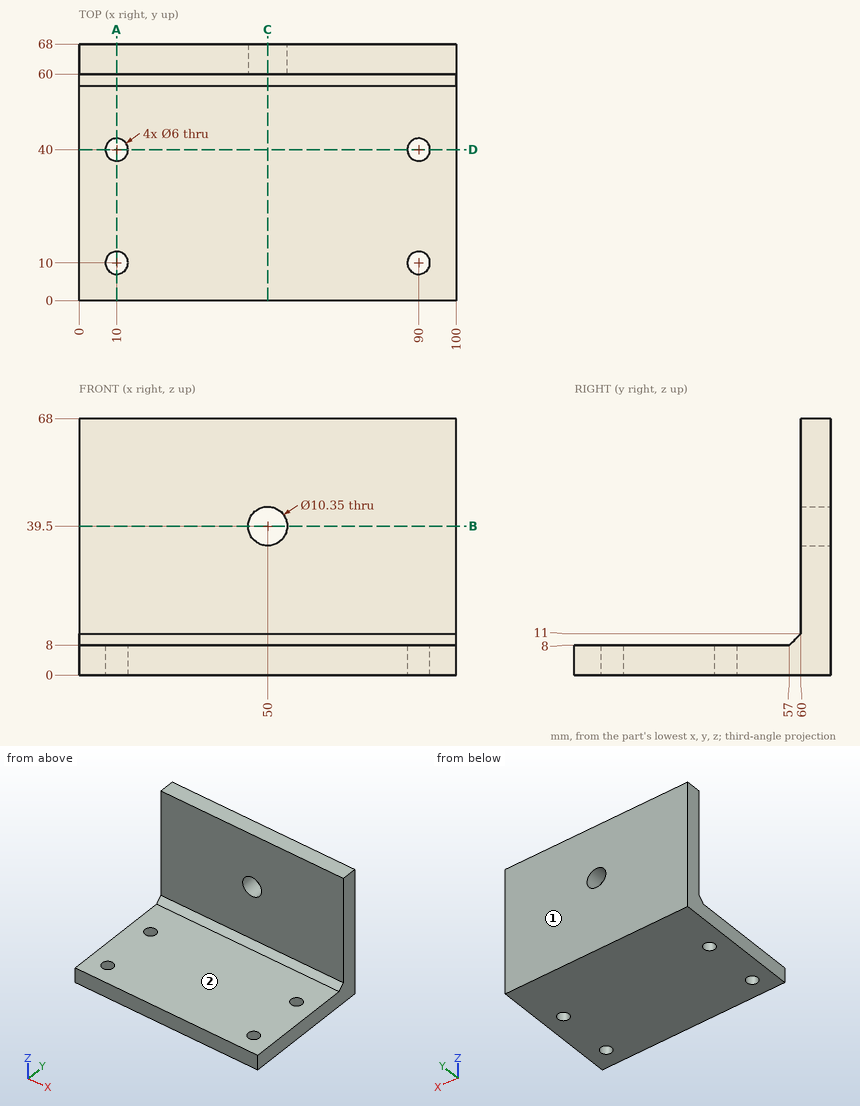
Answer from the drawing. Dimensions are ordinates in mm from the lowest x, y and z of the part. A direction names the side the tool comes from. Coordinates: 2 decimals unless noted, no trailing zeros. Write each loop counter-clockwise with the first axis right and the second up, starting at its lowest first coordinate (ties: lowest second). Pieces come first, ordered by that corner, then holes. Notation, with made-up numbers: (78.25, 62.5) - (114.25, 62.5) arc R24 cw to (114.25, 87.5) - close; hole circle Ø8 at (27, 89.25). An arc over 180 degrees is marked (long way). Return JSON: item names as keys, results as strings. Group by question number.
Q1. Find the intervals of material crossed by line 1 along Y through (x, z) = (90, 2.75); line 2 along X through (y, z) = (63, 39); line 3 along Z through (x, y) = (25, 5), in increasing order. Write a range as [from, to].
Q2. The part is cut by section C-C on x = 50. Write down the section's boundary in (y, z) (3 decimals), and give its area (3 significant figures).
Q3. The part is cut by section B-B on z = 39.5. Write down the section's boundary in (x, y) (3 decimals), and give its area (3 significant figures).
Q4. Flat-ended cylindrical pins translate along their axes: pin 1 Ø10 at (x, z) = (55, 16.5) entering from -Y; pin 2 Ø8 at (x, y) = (90, 10) entering from +Z. Find the tip coordinate at first contact, or state that the pin passes through.
Q5. Which of the six approach directions +Z, -Z, +X, -X, +Y, -Y give full straight-line access (tool end or side, diameter ignored) to the marked faces 1 and 2?
Q6. The part is cut by section A-A on x = 10. Write down the section's boundary in (y, z), and give its area (4 significant figures).
Q7. The part is cut by section D-D on y = 40. Write down the section's boundary in (x, z), and give its area (3 significant figures).
Evaluation:
{
 "1": {"line 1": "y = [0, 7], [13, 37], [43, 68]", "line 2": "x = [0, 44.85], [55.15, 100]", "line 3": "z = [0, 8]"},
 "2": {"outline": "(0, 0) - (68, 0) - (68, 34.325) - (60, 34.325) - (60, 11) - (57, 8) - (0, 8) - close; (60, 44.675) - (68, 44.675) - (68, 68) - (60, 68) - close", "area": "946 mm2"},
 "3": {"outline": "(0, 60) - (44.825, 60) - (44.825, 68) - (0, 68) - close; (55.175, 60) - (100, 60) - (100, 68) - (55.175, 68) - close", "area": "717 mm2"},
 "4": {"pin 1": "stops at y = 60", "pin 2": "stops at z = 8"},
 "5": {"face 1": "+Z, -Z, +X, -X, +Y", "face 2": "+Z, +X, -X, -Y"},
 "6": {"outline": "(0, 0) - (7, 0) - (7, 8) - (0, 8) - close; (13, 0) - (37, 0) - (37, 8) - (13, 8) - close; (43, 0) - (68, 0) - (68, 68) - (60, 68) - (60, 11) - (57, 8) - (43, 8) - close", "area": "932.5 mm2"},
 "7": {"outline": "(0, 0) - (7, 0) - (7, 8) - (0, 8) - close; (13, 0) - (87, 0) - (87, 8) - (13, 8) - close; (93, 0) - (100, 0) - (100, 8) - (93, 8) - close", "area": "704 mm2"}
}
